Here's how the part is built. I have some questions about the finished solid (model axes, mm). Round coordinates to 2 decimals unless told otherwise and drop trailing zeros. Write each loop counter-clockwise with the first axis right and the second up, starting at its lowest first coordinate (ties: lowest second). Pieces come first, ordered by that corner, then holes. Notation, with made-up numbers: (7, -25.5) -> (25, -25.5) arc R18 ccw to (25, -11.5) -> close; hole circle Ø4 at (-20.5, -6). An arc over 180 degrees is marked (long way). Answer in a Markdown table with one row per item. Add a question column.
Autodesk Inventor part; units mm, degrees
ref_plane "YZ Plane" through (0, 0, 0) normal (1, 0, 0) x (0, 1, 0)
ref_plane "XZ Plane" through (0, 0, 0) normal (0, 1, 0) x (-1, 0, 0)
ref_plane "XY Plane" through (0, 0, 0) normal (0, 0, 1) x (1, 0, 0)
sketch "Sketch1" plane through (0, 0, 0) normal (0, 0, 1) x (1, 0, 0)
  line L0 (320, 0) -> (320, 670)
  line L1 (320, 670) -> (-480, 670)
  line L2 (-480, 670) -> (-480, 0)
  circle A0 centre (0, 350) radius 40
  line L3 (320, 0) -> (-480, 0)
  point P0 (0, 0)
  dimension "d14" = 80
  dimension "d15" = 320
  dimension "d17" = 320
  dimension "d26" = 800
  dimension "d27" = 670
extrude "Plate1" add sketch "Sketch1" along normal blind 3
sketch "Sketch3" plane through (0, 0, 3) normal (0, 0, 1) x (1, 0, 0)
  circle A0 centre (0, 405) radius 5
  circle A1 centre (0, 350) radius 40
  point P0 (0, 0)
  dimension "d19" = 10
  dimension "d20" = 55
extrude "Cut1" cut sketch "Sketch3" against normal through all contours A0
pattern_circular "Circular Pattern1" count 6 over 360 about axis through (0, 350, 0) along (0, 0, 1) of "Cut1"
sketch "Sketch4" plane through (0, 0, 3) normal (0, 0, 1) x (1, 0, 0)
  line L0 (100, 650) -> (300, 650) construction
  line L1 (300, 650) -> (300, 630) construction
  line L2 (300, 630) -> (100, 630) construction
  line L3 (100, 630) -> (100, 650) construction
  line L4 (-480, 670) -> (320, 670)
  line L5 (320, 670) -> (320, 0)
  point P0 (0, 0)
  dimension "d28" = 200
  dimension "d29" = 20
  dimension "d30" = 20
  dimension "d31" = 20
mark "Mark2"
sketch "Sketch5" plane through (-480, 670, 3) normal (0, 0, 1) x (1, 0, 0)
  circle A0 centre (72.8, -605.5) radius 44.5
  line L0 (0, -670) -> (0, 0)
  line L1 (800, -670) -> (0, -670)
  dimension "d32" = 72.8
  dimension "d33" = 89
  dimension "d34" = 64.5
extrude "Extrusion1" cut sketch "Sketch5" against normal through all
sketch "Sketch6" plane through (-480, 670, 3) normal (0, 0, 1) x (1, 0, 0)
  circle A0 centre (480, -320) radius 40
  line L0 (480, -320) -> (480, -670) construction
  line L1 (0, -670) -> (800, -670)
  line L2 (390, -535) -> (570, -535) construction
  line L3 (390, -541) -> (570, -541)
  line L4 (570, -529) -> (390, -529)
  arc A1 (390, -529) -> (390, -541) centre (390, -535) ccw
  arc A2 (570, -541) -> (570, -529) centre (570, -535) ccw
  line L5 (390, -635) -> (570, -635) construction
  line L6 (390, -641) -> (570, -641)
  line L7 (570, -629) -> (390, -629)
  arc A3 (390, -629) -> (390, -641) centre (390, -635) ccw
  arc A4 (570, -641) -> (570, -629) centre (570, -635) ccw
  line L8 (480, -535) -> (480, -635) construction
  line L9 (366, -515) -> (594, -515) construction
  line L10 (594, -515) -> (594, -655) construction
  line L11 (594, -655) -> (366, -655) construction
  line L12 (366, -655) -> (366, -515) construction
  line L13 (366, -515) -> (594, -655) construction
  circle A5 centre (366, -515) radius 2.5
  line L14 (442, -515) -> (442, -655) construction
  line L15 (518, -515) -> (518, -655) construction
  circle A6 centre (442, -515) radius 2.5
  circle A7 centre (518, -515) radius 2.5
  circle A8 centre (594, -515) radius 2.5
  circle A9 centre (594, -585) radius 2.5
  circle A10 centre (594, -655) radius 2.5
  circle A11 centre (518, -655) radius 2.5
  circle A12 centre (442, -655) radius 2.5
  circle A13 centre (366, -655) radius 2.5
  circle A14 centre (366, -585) radius 2.5
  point P0 (480, -585)
  dimension "d37" = 180
  dimension "d38" = 12
  dimension "d41" = 100
  dimension "d42" = 85
  dimension "d43" = 228
  dimension "d45" = 5
  dimension "d46" = 140
  dimension "d47" = 76
  dimension "d48" = 76
extrude "Extrusion2" cut sketch "Sketch6" against normal through all contours A1 L4 A2 L3 | A3 L7 A4 L6
equation "\"d2\" = Thickness"
equation "\"BendReliefWidth\" = Thickness"
equation "\"BendReliefDepth\" = 0.5 * Thickness"
equation "\"CornerReliefSize\" = 4 * Thickness"
equation "\"MinimumRemnant\" = 2 * Thickness"
equation "\"TransitionRadius\" = BendRadius"
equation "\"JacobiRadiusSize\" = BendRadius"
equation "\"GapSize\" = Thickness"
properties part number "TRM 016 right board main++" material "AISI 304"
Item 1: I need wall thicknesses on line 1 along Y through (x, z) = (0, 1.3); line 2 along Y through (x, z) = (85, 1.45); line 3 along X through (y, z) = (65.5, 2.5). Which ranges of each line are inside material? Lowest first, please. Write a range as from..to.
Item 2: If we mould it in two halves opening along X, with no side actions, what happens to faces 1 (the cylindrical face through (-5.21, 310.34, 1.48)), 2 (the flat face through (-86, 340, 3))? For each: pulls with the +X half, pulls with the -X half, needs draft (parallel to the pull), parting line crosses it, or undercut.
Item 3: If we section it at D-D on x = 30: Please give me the cut outline in (y, z).
Item 4: For P1, Ø2, axis at x = -82.5, y = 578, coming from the -Z side, with a flat end and sliding along its axis, tell me the tip position at first contact or that it passes through.
Item 5: If we section it at B-B on x = -407.2: Please give me the cut outline in (y, z), then the cut area to 3 significant figures.
Item 6: If we section it at C-C on z = 0.7: Give the number of separate pieces and of enclosed holes in the cut face, then the cut area to 3 significant figures.
Item 7: If we section it at A-A on y = 84: Please give me the cut outline in (x, z).
Results list:
| question | item | result |
|---|---|---|
| 1 | line 1 | 0..29, 41..129, 141..290, 300..310, 390..400, 410..670 |
| 1 | line 2 | 0..29, 41..129, 141..670 |
| 1 | line 3 | -480..-451.69, -362.71..320 |
| 2 | face 1 | undercut |
| 2 | face 2 | needs draft |
| 3 | outline | (0, 0) -> (29, 0) -> (29, 3) -> (0, 3) -> close; (41, 0) -> (129, 0) -> (129, 3) -> (41, 3) -> close; (141, 0) -> (323.54, 0) -> (323.54, 3) -> (141, 3) -> close; (376.46, 0) -> (670, 0) -> (670, 3) -> (376.46, 3) -> close |
| 4 | P1 | z = 0 |
| 5 | outline | (0, 0) -> (20, 0) -> (20, 3) -> (0, 3) -> close; (109, 0) -> (670, 0) -> (670, 3) -> (109, 3) -> close |
| 5 | area | 1,740 mm² |
| 6 | separate pieces | 1 |
| 6 | enclosed holes | 10 |
| 6 | area | 520,000 mm² |
| 7 | outline | (-480, 0) -> (-447.2, 0) -> (-447.2, 3) -> (-480, 3) -> close; (-367.2, 0) -> (320, 0) -> (320, 3) -> (-367.2, 3) -> close |
